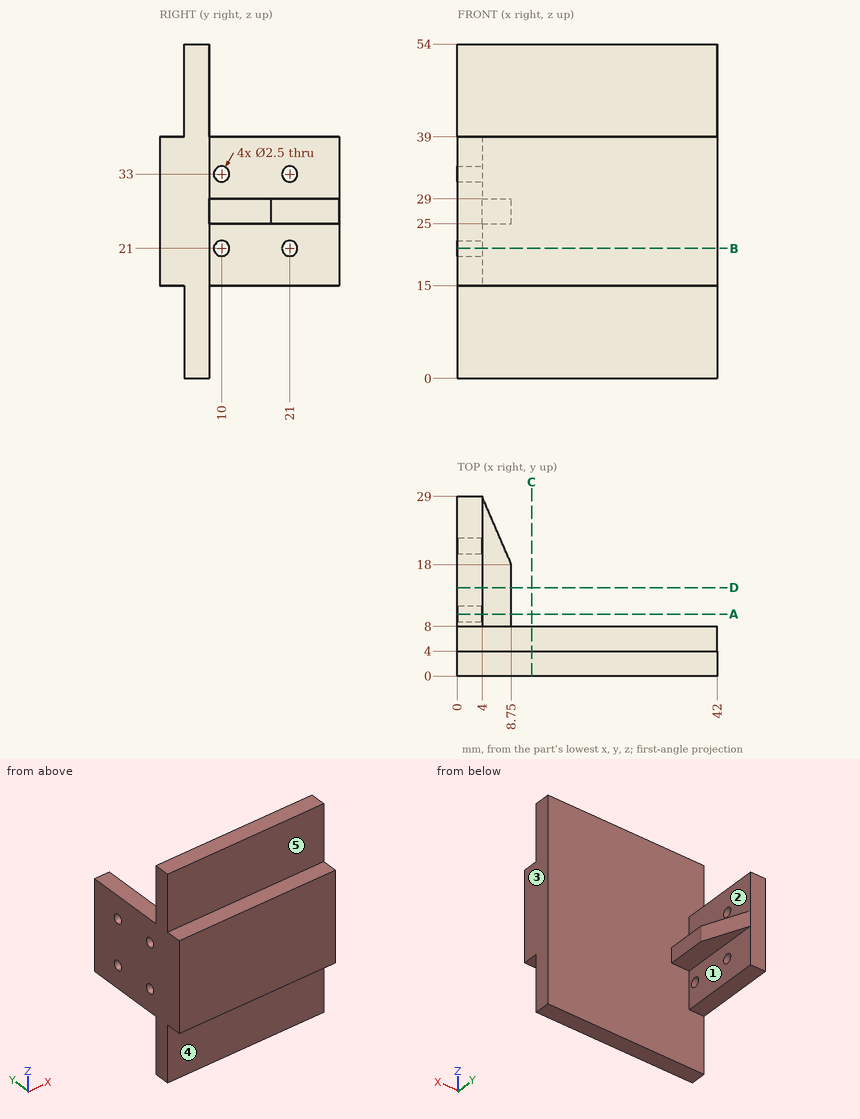
Geometry: see drawing. Coordinates: mm, zero at the bounding-box minimum. A direction names the side the tool comes from. Coordinates: 2 decimals unless noted, no trailing zeros. Loops run counter-clockwise (first coordinate to the right, second up) from the corner with the lowest first, then second, coordinate; pieces in that order, holes last.
Q1. Cut plane C-C (x = 12). Output: boundary loops of the cut face in (y, z), then the cut area to 3 significant figures.
Q2. Cut plane D-D (y = 14.25). Output: boundary loops of the cut face in (x, z), then the cut area to 3 significant figures.
Q3. Cut plane B-B (z = 21). Output: boundary loops of the cut face in (x, y).
Q4. Contact query for flat-ended pins moving along their axis: pin 1 (4 mm diameter, centred on y = 21, z = 21, fed in from +X); pin 2 (2 mm diameter, centred on x = 2.5, y = 17.5, fed in from -Z); pin 3 (4 mm diameter, centred on x = 6.5, y = 16, fed in from -Z); pin 4 (2 mm diameter, centred on y = 10, z = 21, fed in from +X). Output: stop coordinate, or through.
Q5. Set-up query: the marked faces 1, 2, 3, 4 and 5. Return all of +Z, -Z, +X, -X, +Y, -Y with unobstructed straight access to the full face (end or side cutting, diameter ignored); none if empty.
Q6. Material intervals for line 1 (Z direction, x = 2.1, y = 21); line 2 (Y direction, x = 29, z = 24.5); line 3 (Y direction, x = 23, z = 40), sorted ascending.
Q7. Cut plane A-A (y = 10). Output: boundary loops of the cut face in (x, z).
Working result:
1. outline: (0, 15) - (4, 15) - (4, 0) - (8, 0) - (8, 54) - (4, 54) - (4, 39) - (0, 39) - close
1. area: 312 mm2
2. outline: (0, 15) - (4, 15) - (4, 25) - (8.75, 25) - (8.75, 29) - (4, 29) - (4, 39) - (0, 39) - close
2. area: 115 mm2
3. outline: (0, 0) - (42, 0) - (42, 8) - (4, 8) - (4, 8.75) - (0, 8.75) - close; (0, 11.25) - (4, 11.25) - (4, 19.75) - (0, 19.75) - close; (0, 22.25) - (4, 22.25) - (4, 29) - (0, 29) - close
4. pin 1: stops at x = 4
4. pin 2: stops at z = 15
4. pin 3: stops at z = 25
4. pin 4: passes through
5. face 1: -Z, +X, +Y
5. face 2: +Z, +X, +Y
5. face 3: +Z, -Z, +X, +Y, -Y
5. face 4: -Z, +X, -X, -Y
5. face 5: +Z, +X, -X, -Y
6. line 1: z = 15 to 19.75, 22.25 to 31.75, 34.25 to 39
6. line 2: y = 0 to 8
6. line 3: y = 4 to 8
7. outline: (0, 15) - (4, 15) - (4, 19.75) - (0, 19.75) - close; (0, 22.25) - (4, 22.25) - (4, 25) - (8.75, 25) - (8.75, 29) - (4, 29) - (4, 31.75) - (0, 31.75) - close; (0, 34.25) - (4, 34.25) - (4, 39) - (0, 39) - close
